Check sheet for the modelled part. Datum: model origin and axes. Units: mm. Face numbers are marked on the shaded views. A direction names the side the tool comes from. Coordinates: 2 decimals unless noted, no trailing zeros. Write each loop counter-clockwise with the first axis right and the second up, starting at its lowest first coordinate (ties: lowest second). Pieces come first, ordered by that corner, then holes. Notation, with made-up numbers: (22, 43.25) -> (72, 43.25) arc R29 cw to (72, 74.25) -> close; hole circle Ø8 at (23, 43.5). An arc over 180 degrees is marked (long way). One line per item, written item: value. Start each with the question number.
1) Scan lines: line 1 along Y through (x, z) = (0, -6.75); line 2 along X through (y, z) = (10, -3.5); line 3 along X through (y, z) = (10, -6.25). Record each from-to range of solid material in increasing order. Write a range as [from, to].
2) Gauge pin test, flat ends, axial feed: P1, Ø1, axis at x = 2, y = 12.5, coming from the -Z side; P2, Ø1, axis at y = 8, z = -8.5, coming from the +X side. Record the tip position at first contact, or that the pin passes through.
3) Draft check along X on the marked faces 3, 4, 5 and 6. Enter one of: +X half, -X half, draft (parallel to the pull), parting line (faces both ways), or undercut.
4) Sectioned sample at C-C on y = 2.5. Enter the section's corners in (x, z).
5) Sectioned sample at D-D on y = 10. Enter the section's corners in (x, z), plus the area to 3 significant figures.
6) Set-up check for the marked faces 1 and 2: record each of +Z, -Z, +X, -X, +Y, -Y from which the full face is reachable in a straight line by a thin tool's end or side.
7) Sectioned sample at A-A on x = 0. Enter the section's corners in (y, z).
8) Sectioned sample at B-B on z = -4.75. Enter the section's corners in (x, y), plus the area to 3 significant figures.
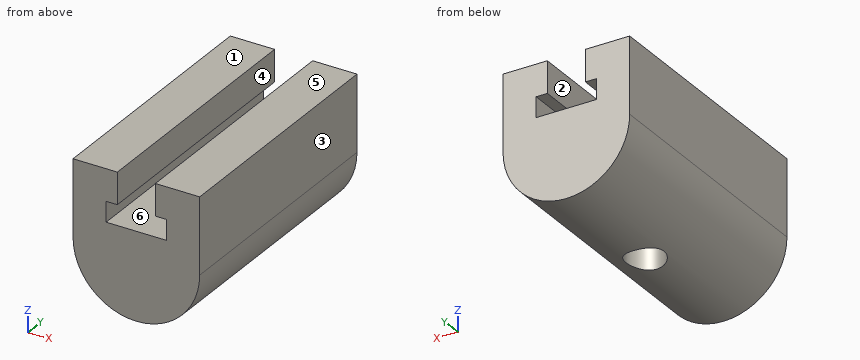
Autodesk Inventor part; units mm, degrees
ref_plane "YZ Plane" through (0, 0, 0) normal (1, 0, 0) x (0, 1, 0)
ref_plane "XZ Plane" through (0, 0, 0) normal (0, 1, 0) x (-1, 0, 0)
ref_plane "XY Plane" through (0, 0, 0) normal (0, 0, 1) x (1, 0, 0)
sketch "Sketch1" plane through (0, 0, 0) normal (0, 1, 0) x (-1, 0, 0)
  line L0 (7, 0) -> (-7, 0)
  line L1 (0, -13.2) -> (0, 2.2)
  line L2 (-5, 0) -> (-5, -6)
  line L3 (5, -6) -> (5, 0)
  line L4 (1.5, 0) -> (1.5, -2.5)
  line L5 (1.5, -2.5) -> (2.3876, -2.5)
  line L6 (2.3876, -2.5) -> (2.3876, -4.1002)
  line L7 (2.3876, -4.1002) -> (0, -4.1002)
  line L8 (-1.5, 0) -> (-1.5, -2.5)
  line L9 (-1.5, -2.5) -> (-2.3876, -2.5)
  line L10 (-2.3876, -2.5) -> (-2.3876, -4.1002)
  line L11 (-2.3876, -4.1002) -> (0, -4.1002)
  line L12 (5, 0) -> (1.5, 0)
  line L13 (-1.5, 0) -> (-5, 0)
  arc A0 (-5, -6) -> (5, -6) centre (0, -6) ccw
  point P0 (0, 0)
  dimension "d0" = 10
  dimension "d1" = 5
  dimension "d3" = 2.3876
  dimension "d4" = 1.6002
  dimension "d5" = 2.5
  dimension "d6" = 1.5
  dimension "d7" = 6
  dimension "d8" = 5
extrude "Extrusion1" add sketch "Sketch1" along normal blind 20 contours L3 A0 L1 L7 L6 L5 L4 L0 | A0 L2 L0 L8 L9 L10 L11 L1
sketch "Sketch2" plane through (-2.3876, 0, -4.1002) normal (0, 0, 1) x (1, 0, 0)
  line L0 (2.3876, 0) -> (2.3876, 20) construction
  line L1 (7.3876, 20) -> (-2.6124, 20)
  circle A0 centre (2.3876, 10) radius 1.5
  dimension "d11" = 3
extrude "Extrusion2" cut sketch "Sketch2" against normal blind 20
equation "\"d1\" = 0.5 * d0"
properties part number "BallBallerina_StopHead"
Answers:
1. line 1: y = [0, 8.5], [11.5, 20]
1. line 2: x = [-5, -2.39], [2.39, 5]
1. line 3: x = [-4.99, -1.5], [1.5, 4.99]
2. P1: stops at z = -10.77
2. P2: stops at x = 4.58
3. face 3: +X half
3. face 4: undercut
3. face 5: draft
3. face 6: undercut
4. outline: (-5, -6) arc R5 ccw to (5, -6) -> (5, 0) -> (1.5, 0) -> (1.5, -2.5) -> (2.39, -2.5) -> (2.39, -4.1) -> (-2.39, -4.1) -> (-2.39, -2.5) -> (-1.5, -2.5) -> (-1.5, 0) -> (-5, 0) -> close
5. outline: (-5, -6) arc R5 ccw to (-1.5, -10.77) -> (-1.5, -4.1) -> (-2.39, -4.1) -> (-2.39, -2.5) -> (-1.5, -2.5) -> (-1.5, 0) -> (-5, 0) -> close; (1.5, -10.77) arc R5 ccw to (5, -6) -> (5, 0) -> (1.5, 0) -> (1.5, -2.5) -> (2.39, -2.5) -> (2.39, -4.1) -> (1.5, -4.1) -> close
5. area: 63.7 mm2
6. face 1: +Z, +X, -X, +Y, -Y
6. face 2: +Z, +Y, -Y
7. outline: (0, -11) -> (8.5, -11) -> (8.5, -4.1) -> (0, -4.1) -> close; (11.5, -11) -> (20, -11) -> (20, -4.1) -> (11.5, -4.1) -> close
8. outline: (-5, 0) -> (5, 0) -> (5, 20) -> (-5, 20) -> close; hole circle Ø3 at (0, 10)
8. area: 193 mm2
